For this review, take the finished solid that the model builds, in its own axes (mm). Face numbers are marked on the shaded views. A direction names the side the tool comes from. Coordinates: 2 decimals unless noted, no trailing zeros. Loops run counter-clockwise (first coordinate to the right, second up) from the corner with the lowest first, then second, coordinate; pieces in that order, holes last. Notation, with made-up numbers: M -1,2.5 L 7,2.5 A16 cw 7,26.5 Z; hole C -5.75,46 d5. An arc over 180 degrees is marked long. Answer as a JSON object with one key per item and string values. Group by question number.
Item 1: Add section B-B (z = 5). State the section outline as (x, y) points.
Item 2: Mouldability with a two-part tool opening along X and no side actions: class the marked faces 1, 2 and 3 as +X half, -X half, draft (parallel to the pull), parting line (faces both ways), or undercut.
Item 3: Wall thickness on L1, parallel to X at y = -19, z = 8; L2, parallel to X at y = -22.8, z = 5; L3, parallel to Y at x = -4, z = 9.25: over which ranges is each line inside the solid? List them lowest first. Write a range as from..to.
Item 4: Tool access review of the marked faces 4, 5, 6, 7 and 8: name each direction out of +Z, -Z, +X, -X, +Y, -Y from which nothing blocks a thin tool from reaching the whole face with its end or side.
Item 5: Add section C-C (y = -7). State the section outline as (x, z) points.
Item 6: Insertion check: pin 1 (1.5 mm diameter, centred on y = -15.5, z = 5.5, fed in from -X); pin 2 (3 mm diameter, centred on y = -17.5, z = 2.5, fed in from +X); pin 3 (3 mm diameter, centred on x = -8.5, z = 1.5, fed in from +Y); pin 4 (2.5 mm diameter, centred on x = 0, z = 5, fed in from -Y). Each pin has a flat end and moves straight along its axis. Give the tip position at first contact, or say it passes through.
Item 7: Add section A-A (x = 0). State the section outline as (y, z) points, then the cut area to 3 significant figures.
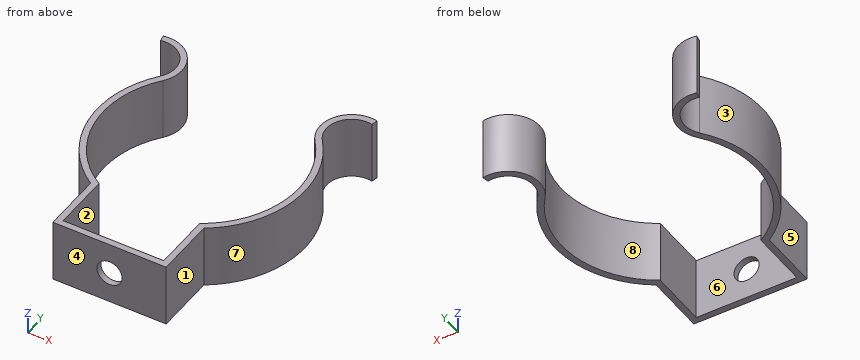
from build123d import *

# Parameters (mm, degrees)
BOSS_EXTRUDE1_DEPTH = 10
SKETCH2_R           = 2
CUT_EXTRUDE1_DEPTH  = 10


with BuildPart() as part:
    # Sketch1 → Boss-Extrude1 (new body)
    with BuildSketch(Plane.XY):
        with BuildLine():
            Line((8, -22.5), (8, -13.275918047))
            ThreePointArc((8, -13.275918047), (15.259032291, -2.722486649), (12.097560976, 9.690150589))
            ThreePointArc((12.097560976, 9.690150589), (11.733206084, 15.422625974), (17, 17.714985104))
            Line((17, 17.714985104), (16.8, 16.735189206))
            ThreePointArc((16.8, 16.735189206), (12.586564868, 14.901301903), (12.87804878, 10.315321595))
            ThreePointArc((12.87804878, 10.315321595), (16.291198361, -2.616649759), (9, -13.829316686))
            Line((9, -13.829316686), (9, -23.5))
            Line((9, -23.5), (-9, -23.5))
            Line((-9, -23.5), (-9, -13.829316686))
            ThreePointArc((-9, -13.829316686), (-16.291198361, -2.616649759), (-12.87804878, 10.315321595))
            ThreePointArc((-12.87804878, 10.315321595), (-12.586564868, 14.901301903), (-16.8, 16.735189206))
            Line((-16.8, 16.735189206), (-17, 17.714985104))
            ThreePointArc((-17, 17.714985104), (-11.733206084, 15.422625974), (-12.097560976, 9.690150589))
            ThreePointArc((-12.097560976, 9.690150589), (-15.259032291, -2.722486649), (-8, -13.275918047))
            Line((-8, -13.275918047), (-8, -22.5))
            Line((-8, -22.5), (8, -22.5))
        make_face()
    extrude(amount=BOSS_EXTRUDE1_DEPTH)

    # Sketch2 → Cut-Extrude1 (cut)
    with BuildSketch(Plane(origin=(0, -22.5, 0), x_dir=(1, 0, 0), z_dir=(0, 1, 0))):
        with Locations(Location((0, -5, 0), (0, 0, 270))):
            Circle(SKETCH2_R)
    extrude(amount=-CUT_EXTRUDE1_DEPTH, mode=Mode.SUBTRACT)


solid = part.part
From the geometry:
{
 "1": {"outline": "M -17,17.71 L -16.8,16.74 A4 cw -12.88,10.32 A16.5 ccw -9,-13.83 L -9,-23.5 L -2,-23.5 L -2,-22.5 L -8,-22.5 L -8,-13.28 A15.5 cw -12.1,9.69 A5 ccw Z; M 2,-23.5 L 9,-23.5 L 9,-13.83 A16.5 ccw 12.88,10.32 A4 cw 16.8,16.74 L 17,17.71 A5 ccw 12.1,9.69 A15.5 cw 8,-13.28 L 8,-22.5 L 2,-22.5 Z"},
 "2": {"face 1": "+X half", "face 2": "undercut", "face 3": "-X half"},
 "3": {"L1": "x = -9..-8, 8..9", "L2": "x = -9..-2, 2..9", "L3": "y = -23.5..-22.5"},
 "4": {"face 4": "+Z, -Z, +X, -X, -Y", "face 5": "+Z, -Z, -X, -Y", "face 6": "+Z, -Z, +Y", "face 7": "+Z, -Z, +X", "face 8": "+Z, -Z"},
 "5": {"outline": "M -14.94,0 L -13.83,0 L -13.83,10 L -14.94,10 Z; M 13.83,0 L 14.94,0 L 14.94,10 L 13.83,10 Z"},
 "6": {"pin 1": "stops at x = -9", "pin 2": "stops at x = 9", "pin 3": "stops at y = -11.84", "pin 4": "passes through"},
 "7": {"outline": "M -23.5,0 L -22.5,0 L -22.5,3 L -23.5,3 Z; M -23.5,7 L -22.5,7 L -22.5,10 L -23.5,10 Z", "area": "6.00 mm²"}
}
